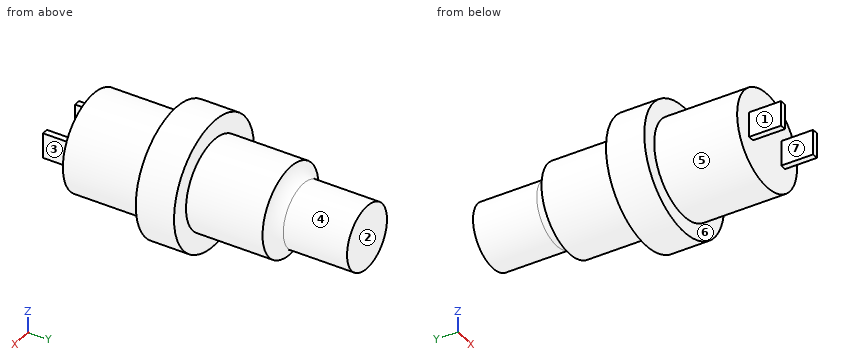
from build123d import *

# Parameters (mm, degrees)
SKETCH_1_R      = 3.75
EXTRUDE_1_DEPTH = 6.5
SKETCH_2_R      = 5
EXTRUDE_2_DEPTH = 3
SKETCH_3_R      = 3.5
EXTRUDE_3_DEPTH = 6
SKETCH_4_R      = 2.5
EXTRUDE_4_DEPTH = 6
FILLET_1_R      = 1
SKETCH_5_W      = 0.48356718
SKETCH_5_H      = 1.971466194
EXTRUDE_5_DEPTH = 2.5


with BuildPart() as part:
    # Эскиз1 → Бобышка-Вытянуть1 (new body)
    with BuildSketch(Plane(origin=(0, 0, 0), x_dir=(1, 0, 0), z_dir=(0, 1, 0))):
        with Locations(Location((0, 0, 0), (0, 0, 90))):
            Circle(SKETCH_1_R)
    extrude(amount=EXTRUDE_1_DEPTH)

    # Эскиз2 → Бобышка-Вытянуть2 (add)
    with BuildSketch(Plane(origin=(0, 6.5, 0), x_dir=(1, 0, 0), z_dir=(0, 1, 0))):
        with Locations(Location((0, 0, 0), (0, 0, 270))):
            Circle(SKETCH_2_R)
    extrude(amount=EXTRUDE_2_DEPTH)

    # Эскиз3 → Бобышка-Вытянуть3 (add)
    with BuildSketch(Plane(origin=(0, 9.5, 0), x_dir=(1, 0, 0), z_dir=(0, 1, 0))):
        with Locations(Location((0, 0, 0), (0, 0, 270))):
            Circle(SKETCH_3_R)
    extrude(amount=EXTRUDE_3_DEPTH)

    # Эскиз4 → Бобышка-Вытянуть4 (add)
    with BuildSketch(Plane(origin=(0, 15.5, 0), x_dir=(1, 0, 0), z_dir=(0, 1, 0))):
        with Locations(Location((0, 0, 0), (0, 0, 270))):
            Circle(SKETCH_4_R)
    extrude(amount=EXTRUDE_4_DEPTH)

    # Скругление1
    fillet_1_edges = [part.edges().sort_by_distance(p)[0] for p in [
        (0, 15.5, -2.5),
    ]]
    fillet(fillet_1_edges, radius=FILLET_1_R - 0.0001)  # a hair under: the kernel refuses the full size

    # Эскиз5 → Бобышка-Вытянуть5 (add)
    with BuildSketch(Plane.XZ):
        with Locations((2.00821641, 0)):
            Rectangle(SKETCH_5_W, SKETCH_5_H)
        with Locations((-2.00821641, 0)):
            Rectangle(SKETCH_5_W, SKETCH_5_H)
    extrude(amount=EXTRUDE_5_DEPTH)


solid = part.part
Design review of the part built by this model. Coordinates are the model's own, in mm. Face numbers are marked on the shaded views. A direction names the side the tool comes from. Give positions to 0.01 mm unless a question says otherwise; leave off trailing zeros. Loops run counter-clockwise (first coordinate to the right, second up) from the corner with the lowest first, then second, coordinate; pieces in that order, holes last. Notation, with made-up numbers: M 29.5,27.25 L 55.5,27.25 A29 ccw 55.5,66.25 Z; hole C 35.5,42 d8. An arc over 180 degrees is marked long. One line per question, with ' | ' between items. Start each with the question number.
1. For the marked faces 1, 2, 3 and 4, list the 3-axis set-ups (+Z, -Z, +X, -X, +Y, -Y) from which the entire face can be reached by the end or side of a thin tool; tool diameter is ignored.
2. Add section C-C (y = 4.75). Write out the cut boundary in (x, z).
3. The part is to be moulded in two halves that separate along X. For the marked faces 5, 6 and 7, say which applies: released by +X, released by -X, zero draft, split by the parting line, or undercut.
4. Add section B-B (y = 7.5). Write out the cut boundary in (x, z), plus the area to 3 significant figures.
5. To check wall thickness, follow L1, parallel to Y at x = -0.75, z = 2.25; L2, parallel to Y at x = 0.25, z = 4.75; L3, parallel to Z at x = -0.25, y = 16.75. State the ranges of each line that lie inside material, in increasing order.
6. Insertion check: P1, Ø4, axis at y = 18.5, z = 0.5, coming from the +X side; P2, Ø3, axis at y = 8.5, z = 2.5, coming from the +X side; P3, Ø1.6, axis at y = -1.5, z = 0, coming from the -X side. Each pin has a flat end and moves straight along its axis. Give the tip position at first contact, or say it passes through.
Worked out:
1) face 1: +Z, -Z, -X, -Y | face 2: +Z, -Z, +X, -X, +Y | face 3: +Z, -Z, +X, -Y | face 4: +Y
2) outline: C 0,0 d7.5
3) face 5: split by the parting line | face 6: zero draft | face 7: undercut
4) outline: C 0,0 d10 | area: 78.5 mm²
5) L1: y = 0 to 21.5 | L2: y = 6.5 to 9.5 | L3: z = -2.49 to 2.49
6) P1: stops at x = 2.5 | P2: stops at x = 4.9 | P3: stops at x = -2.25
